```python
from build123d import *

# Parameters (mm, degrees)
BOSS_EXTRUDE1_DEPTH     = 3
CUT_EXTRUDE1_DEPTH      = 10
CUT_EXTRUDE1_DEPTH_BACK = 10
SKETCH2_R               = 1.375
CUT_EXTRUDE2_DEPTH      = 10
CUT_EXTRUDE2_DEPTH_BACK = 10
SKETCH4_R               = 1.6086033
SKETCH4_R_2             = 1.6
SKETCH4_R_3             = 1.600016576
SKETCH4_R_4             = 1.599999999
CUT_EXTRUDE3_DEPTH      = 5
CUT_EXTRUDE3_DEPTH_BACK = 5
SKETCH5_R               = 2
SKETCH5_R_2             = 1.996887868
CHAMFER1_SIZE           = 25
CHAMFER1_SIZE2          = 34.359213547
CHAMFER1_EDGE_2_SIZE    = 25
CHAMFER1_EDGE_2_SIZE2   = 34.359213547
CUT_EXTRUDE4_DEPTH      = 10
CUT_EXTRUDE4_DEPTH_BACK = 10
SKETCH6_R               = 1.631965818
SKETCH6_R_2             = 1.621215412
SKETCH6_R_3             = 1.651492617
SKETCH6_R_4             = 1.62625173
CUT_EXTRUDE5_DEPTH      = 10
CUT_EXTRUDE5_DEPTH_BACK = 10
SKETCH7_R               = 1.35
CUT_EXTRUDE6_DEPTH      = 10
CUT_EXTRUDE6_DEPTH_BACK = 10
SKETCH8_R               = 2


with BuildPart() as part:
    # Sketch1 → Boss-Extrude1 (new body)
    with BuildSketch(Plane(origin=(0, 0, 0), x_dir=(1, 0, 0), z_dir=(0, 1, 0))):
        Polygon((-60, 15), (-60, 0), (60, 0), (60, 15), (37.6, 15), (37.6, 40.3), (60, 40.3), (60, 70), (40, 150), (-40, 150), (-60, 70), (-60, 40.3), (-37.6, 40.3), (-37.6, 15), align=None)
    extrude(amount=BOSS_EXTRUDE1_DEPTH)

    # Sketch2 → Cut-Extrude1 (cut, two sides: drawn at the far end of the back side and taken through both)
    with BuildSketch(Plane(origin=(0, 3, 0), x_dir=(1, 0, 0), z_dir=(0, 1, 0)).offset(-CUT_EXTRUDE1_DEPTH_BACK)):
        with Locations(Location((-31.3, 43, 0), (0, 0, 270))):
            Circle(SKETCH2_R)
        with Locations(Location((-6.3, 43, 0), (0, 0, 270))):
            Circle(SKETCH2_R)
        with Locations(Location((-6.3, 12, 0), (0, 0, 270))):
            Circle(SKETCH2_R)
        with Locations(Location((-31.3, 12, 0), (0, 0, 270))):
            Circle(SKETCH2_R)
        with Locations(Location((6.3, 43, 0), (0, 0, 270))):
            Circle(SKETCH2_R)
        with Locations(Location((31.3, 43, 0), (0, 0, 270))):
            Circle(SKETCH2_R)
        with Locations(Location((31.3, 12, 0), (0, 0, 270))):
            Circle(SKETCH2_R)
        with Locations(Location((6.3, 12, 0), (0, 0, 270))):
            Circle(SKETCH2_R)
    extrude(amount=CUT_EXTRUDE1_DEPTH + CUT_EXTRUDE1_DEPTH_BACK, mode=Mode.SUBTRACT)

    # Sketch4 → Cut-Extrude2 (cut, two sides: drawn at the far end of the back side and taken through both)
    with BuildSketch(Plane(origin=(0, 3, 0), x_dir=(1, 0, 0), z_dir=(0, 1, 0)).offset(-CUT_EXTRUDE2_DEPTH_BACK)):
        with Locations(Location((-22.548030216, 82.366514772, 0), (0, 0, 270))):
            Circle(SKETCH4_R)
        with Locations(Location((-7.372652758, 82.375044524, 0), (0, 0, 270))):
            Circle(SKETCH4_R_2)
        with Locations(Location((22.726359118, 82.375056093, 0), (0, 0, 270))):
            Circle(SKETCH4_R_3)
        with Locations(Location((7.549847242, 82.375044524, 0), (0, 0, 270))):
            Circle(SKETCH4_R_4)
    extrude(amount=CUT_EXTRUDE2_DEPTH + CUT_EXTRUDE2_DEPTH_BACK, mode=Mode.SUBTRACT)

    # Sketch5 → Cut-Extrude3 (cut, two sides: drawn at the far end of the back side and taken through both)
    with BuildSketch(Plane(origin=(0, 3, 0), x_dir=(1, 0, 0), z_dir=(0, 1, 0)).offset(-CUT_EXTRUDE3_DEPTH_BACK)):
        with Locations(Location((-51.988593255, 44.648942023, 0), (0, 0, 270))):
            Circle(SKETCH5_R)
        with Locations(Location((-40.988593255, 44.648942023, 0), (0, 0, 270))):
            Circle(SKETCH5_R)
        with Locations(Location((-51.988593255, 10.65981673, 0), (0, 0, 270))):
            Circle(SKETCH5_R)
        with Locations(Location((-40.988593255, 10.65981673, 0), (0, 0, 270))):
            Circle(SKETCH5_R)
        with Locations(Location((41.011406745, 10.65981673, 0), (0, 0, 270))):
            Circle(SKETCH5_R)
        with Locations(Location((52.011406745, 10.65981673, 0), (0, 0, 270))):
            Circle(SKETCH5_R)
        with Locations(Location((52.011406745, 44.648942023, 0), (0, 0, 270))):
            Circle(SKETCH5_R)
        with Locations(Location((41.01131511, 44.652052806, 0), (0, 0, 270))):
            Circle(SKETCH5_R_2)
    extrude(amount=CUT_EXTRUDE3_DEPTH + CUT_EXTRUDE3_DEPTH_BACK, mode=Mode.SUBTRACT)

    # Chamfer1
    chamfer1_edges = [part.edges().sort_by_distance(p)[0] for p in [
        (-40, 1.5, -150),
    ]]
    chamfer1_side = [part.faces().sort_by_distance(p)[0] for p in [
        (0, 1.5, -150),
    ]]
    chamfer(chamfer1_edges, length=CHAMFER1_SIZE, length2=CHAMFER1_SIZE2, reference=chamfer1_side[0])

    # Chamfer1 edge 2
    chamfer1_edge_2_edges = [part.edges().sort_by_distance(p)[0] for p in [
        (40, 1.5, -150),
    ]]
    chamfer1_edge_2_side = [part.faces().sort_by_distance(p)[0] for p in [
        (0, 1.5, -150),
    ]]
    chamfer(chamfer1_edge_2_edges, length=CHAMFER1_EDGE_2_SIZE, length2=CHAMFER1_EDGE_2_SIZE2, reference=chamfer1_edge_2_side[0])

    # Sketch6 → Cut-Extrude4 (cut, two sides: drawn at the far end of the back side and taken through both)
    with BuildSketch(Plane(origin=(0, 3, 0), x_dir=(1, 0, 0), z_dir=(0, 1, 0)).offset(-CUT_EXTRUDE4_DEPTH_BACK)):
        with Locations(Location((-40.900357492, 106.752555334, 0), (0, 0, 270))):
            Circle(SKETCH6_R)
        with Locations(Location((8.961819516, 105.164972563, 0), (0, 0, 270))):
            Circle(SKETCH6_R_2)
        with Locations(Location((-7.264004675, 55.319530138, 0), (0, 0, 270))):
            Circle(SKETCH6_R_3)
        with Locations(Location((-34.862659576, 55.442184264, 0), (0, 0, 270))):
            Circle(SKETCH6_R_4)
    extrude(amount=CUT_EXTRUDE4_DEPTH + CUT_EXTRUDE4_DEPTH_BACK, mode=Mode.SUBTRACT)

    # Sketch7 → Cut-Extrude5 (cut, two sides: drawn at the far end of the back side and taken through both)
    with BuildSketch(Plane(origin=(0, 3, 0), x_dir=(1, 0, 0), z_dir=(0, 1, 0)).offset(-CUT_EXTRUDE5_DEPTH_BACK)):
        with Locations(Location((18.097012052, 115.64214419, 0), (0, 0, 270))):
            Circle(SKETCH7_R)
        with Locations(Location((41.097012052, 115.64214419, 0), (0, 0, 270))):
            Circle(SKETCH7_R)
        with Locations(Location((18.097012052, 57.64214419, 0), (0, 0, 270))):
            Circle(SKETCH7_R)
        with Locations(Location((41.097012052, 57.64214419, 0), (0, 0, 270))):
            Circle(SKETCH7_R)
    extrude(amount=CUT_EXTRUDE5_DEPTH + CUT_EXTRUDE5_DEPTH_BACK, mode=Mode.SUBTRACT)

    # Sketch8 → Cut-Extrude6 (cut, two sides: drawn at the far end of the back side and taken through both)
    with BuildSketch(Plane.XZ.offset(-CUT_EXTRUDE6_DEPTH_BACK)):
        with Locations(Location((13.75, -135, 0), (0, 0, 90))):
            Circle(SKETCH8_R)
        with Locations(Location((-13.75, -135, 0), (0, 0, 90))):
            Circle(SKETCH8_R)
    extrude(amount=CUT_EXTRUDE6_DEPTH + CUT_EXTRUDE6_DEPTH_BACK, mode=Mode.SUBTRACT)


solid = part.part
```
Read the model definition and answer for the solid it produces. Units are mm, in the model's axes. A direction names the side the tool comes from. Coordinates: 2 decimals unless noted, no trailing zeros. Loops run counter-clockwise (first coordinate to the right, second up) from the corner with the lowest first, then second, coordinate; pieces in that order, holes last.
(1) A tool of negligible diameter and unlimited length cuts with its end or side. For faces 1 (the face through (-49, 1, -15)), 2 (the face through (37.6, 1, -27)), 3 (the face through (50.06, 1.48, -11.09)), from which of +Z, -Z, +X, -X, +Y, -Y can it reach the whole face along a straight path? Write none if from no direction.
Solution:
face 1: -X, +Y, -Y
face 2: +X, +Y, -Y
face 3: +Y, -Y
(2) Flat-ended cylindrical pins translate along their axes: pin 1 Ø1.6 at (x, z) = (18.1, -115.64) entering from +Y; pin 2 Ø1.5 at (x, y) = (-47.5, 1) entering from -Z; pin 3 Ø0.9 at (y, z) = (1.5, -22) entering from +X. Find the tip coordinate at first contact, or state that the pin passes through.
Solution:
pin 1: passes through
pin 2: stops at z = -118.25
pin 3: stops at x = 37.6
(3) The part is cut by section A-A (z = -135). Determine the outline of the cut face in (x, y), and give its area (3 significant figures).
Solution:
outline: (-30, 0) - (-15.75, 0) - (-15.75, 3) - (-30, 3) - close; (-11.75, 0) - (11.75, 0) - (11.75, 3) - (-11.75, 3) - close; (15.75, 0) - (30, 0) - (30, 3) - (15.75, 3) - close
area: 156 mm2
(4) The part is cut by section B-B (y = 1.45). Count the separate pieces of the cut face and the enclosed holes in it, and give its area (3 significant figures).
Solution:
separate pieces: 1
enclosed holes: 30
area: 14,200 mm2
(5) Consider line 1 along Z through (x, y) = (31.3, 1.7) (3 decimals); line 2 along Z through (x, y) = (-7.5, 0.5); line 3 along X through (y, z) = (1.4, -35.5). Determine where each line is inside the solid, lowest interval first.
Solution:
line 1: z = -133.7 to -44.375, -41.625 to -13.375, -10.625 to 0
line 2: z = -150 to -83.97, -80.78 to -56.95, -53.68 to -43.67, -42.33 to -12.67, -11.33 to 0
line 3: x = -37.6 to 37.6
(6) The part is cut by section C-C (z = -26). Determine the outline of the cut face in (x, y).
Solution:
outline: (-37.6, 0) - (37.6, 0) - (37.6, 3) - (-37.6, 3) - close
(7) The mould has two halves that part along Z. Classify faces 4 (the face through (-60, 1, -8)), 5 (the face through (-1, 1, 0)), 6 (the face through (-53.206, 1.479, -46.236)), 7 (the face through (-34.374, 1.479, -53.891)): released by +Z, released by -Z, zero draft, split by the parting line, or undercut.
Solution:
face 4: zero draft
face 5: released by +Z
face 6: undercut
face 7: undercut
